For this review, take the finished solid that the model builds, in its own axes (mm). A direction names the side the tool comes from. Round coordinates to 2 decimals unless told otherwise and drop trailing zeros. Write each loop counter-clockwise with the first axis right and the second up, starting at its lowest first coordinate (ties: lowest second). Pieces come first, ordered by that corner, then holes. Notation, with made-up numbers: M -21.75,-24.75 L 37.25,-24.75 A26 ccw 37.25,4.25 Z; hole C 26,53 d5. An arc over 180 degrees is marked long. Answer in a Markdown table with one row per item.
```python
from build123d import *

# Parameters (mm, degrees)
MAIN_BODY_DEPTH          = 2.6
SKETCH4_W                = 17
SKETCH4_H                = 2.5
FLANGES_DEPTH            = 20.5
SKETCH5_R                = 2
DRILL_HOLD_EXTRUDE_DEPTH = 1.4
SKETCH2_R                = 3.2
SKETCH2_R_2              = 3.15
SKETCH2_R_3              = 1.5
SKETCH2_R_4              = 2.55
SCREW_HOLES_DEPTH        = 21.5
SCREW_HOLES_DEPTH_BACK   = 3.6
FLANGE_FILLET_R          = 2
SKETCH6_W                = 1.5
SKETCH6_H                = 11
FLANGE_NOTCHES_DEPTH     = 26
MAIN_LOWER_BODY_FILLET_R = 2


with BuildPart() as part:
    # Sketch1 → Main Body (new body)
    with BuildSketch(Plane(origin=(0, 0, 0), x_dir=(1, 0, 0), z_dir=(0, 1, 0))):
        with BuildLine():
            Line((11.7, -23.5), (32, -23.5))
            Line((32, -23.5), (32, 13.5))
            ThreePointArc((32, 13.5), (29.071067812, 20.571067812), (22, 23.5))
            Line((22, 23.5), (-22, 23.5))
            ThreePointArc((-22, 23.5), (-29.071067812, 20.571067812), (-32, 13.5))
            Line((-32, 13.5), (-32, -23.5))
            Line((-32, -23.5), (-12, -23.5))
            Line((-12, -23.5), (-12, -46))
            Line((-12, -46), (11.7, -46))
            Line((11.7, -46), (11.7, -23.5))
        make_face()
    extrude(amount=MAIN_BODY_DEPTH)

    # Sketch4 → Flanges (add)
    with BuildSketch(Plane(origin=(0, 2.6, 0), x_dir=(1, 0, 0), z_dir=(0, 1, 0))):
        with Locations((-23.5, -22.25)):
            Rectangle(SKETCH4_W, SKETCH4_H)
        with Locations((23.5, -22.25)):
            Rectangle(SKETCH4_W, SKETCH4_H)
    extrude(amount=FLANGES_DEPTH)

    # Sketch5 → Drill hold extrude (add)
    with BuildSketch(Plane(origin=(0, 2.6, 0), x_dir=(1, 0, 0), z_dir=(0, 1, 0))):
        with Locations((19, -9.3)):
            Circle(SKETCH5_R)
        with Locations((1.5, 9.3)):
            Circle(SKETCH5_R)
    extrude(amount=DRILL_HOLD_EXTRUDE_DEPTH)

    # Sketch2 → Screw holes (cut, two sides)
    with BuildSketch(Plane(origin=(0, 2.6, 0), x_dir=(1, 0, 0), z_dir=(0, 1, 0))) as screw_holes_sk:
        with Locations((-20.1, 15.8)):
            Circle(SKETCH2_R)
        with Locations((20, 16)):
            Circle(SKETCH2_R_2)
        with Locations((1.5, 9.3)):
            Circle(SKETCH2_R_3)
        with Locations((-23.6, -0.5)):
            Circle(SKETCH2_R_3)
        with Locations((-9.5, -0.5)):
            Circle(SKETCH2_R_3)
        with Locations((19, -9.3)):
            Circle(SKETCH2_R_3)
        with Locations((0.7, -31.3)):
            Circle(SKETCH2_R_4)
    extrude(amount=SCREW_HOLES_DEPTH, mode=Mode.SUBTRACT)
    extrude(screw_holes_sk.sketch, amount=-SCREW_HOLES_DEPTH_BACK, mode=Mode.SUBTRACT)

    # Flange Fillet
    flange_fillet_edges = [part.edges().sort_by_distance(p)[0] for p in [
        (-32, 23.1, 22.25),
        (-15, 23.1, 22.25),
        (32, 23.1, 22.25),
        (15, 23.1, 22.25),
    ]]
    fillet(flange_fillet_edges, radius=FLANGE_FILLET_R)

    # Sketch6 → Flange Notches (cut, through all)
    with BuildSketch(Plane(origin=(0, 0, 21), x_dir=(-1, 0, 0), z_dir=(0, 0, -1))):
        with Locations((-20.75, 17.6)):
            Rectangle(SKETCH6_W, SKETCH6_H)
        with Locations((20.75, 17.6)):
            Rectangle(SKETCH6_W, SKETCH6_H)
    extrude(amount=-FLANGE_NOTCHES_DEPTH, mode=Mode.SUBTRACT)

    # Main lower body Fillet
    main_lower_body_fillet_edges = [part.edges().sort_by_distance(p)[0] for p in [
        (11.7, 1.3, 46),
        (-12, 1.3, 46),
    ]]
    fillet(main_lower_body_fillet_edges, radius=MAIN_LOWER_BODY_FILLET_R)


solid = part.part
```
Q1. Machinability: for faces 5 (the face through (17.526, 3.29, 7.948)), 6 (the face through (11.7, 1, 34)), 7 (the face through (21.5, 18, 22)), 8 (the face through (1.175, 2.028, -7.836)), which of the approach directions +Z, -Z, +X, -X, +Y, -Y give a long, thin tool a straight path to every point of the face, cutting with its end or side? Answer none if there is none.
Found:
| item | result |
|---|---|
| face 5 | +Y |
| face 6 | +Z, +X, +Y, -Y |
| face 7 | +Z, -Z, +Y |
| face 8 | +Y, -Y |
Q2. Take a section at A-A (y = 8.25). State the section outline as (x, z) points, then the cut area to 3 significant figures.
Found:
| item | result |
|---|---|
| outline | M -32,21 L -15,21 L -15,23.5 L -32,23.5 Z; M 15,21 L 32,21 L 32,23.5 L 15,23.5 Z |
| area | 85.0 mm² |
Q3. Take a section at B-B (y = 18). State the section outline as (x, z) points, then the cut area to 3 significant figures.
Found:
| item | result |
|---|---|
| outline | M -32,21 L -21.5,21 L -21.5,23.5 L -32,23.5 Z; M -20,21 L -15,21 L -15,23.5 L -20,23.5 Z; M 15,21 L 20,21 L 20,23.5 L 15,23.5 Z; M 21.5,21 L 32,21 L 32,23.5 L 21.5,23.5 Z |
| area | 77.5 mm² |
Q4. For probe 1 along Z at (x, y) = (19, 3.05); probe 2 along X at (y, z) = (2, 0.5); probe 3 along Z at (x, y) = (1.5, 2.85), list the stretches that pass through material, from the lowest coordinate up.
Found:
| item | result |
|---|---|
| probe 1 | 7.3 to 7.8, 10.8 to 11.3, 21 to 23.5 |
| probe 2 | -32 to -25.1, -22.1 to -11, -8 to 32 |
| probe 3 | -11.3 to -10.8, -7.8 to -7.3 |
Q5. Take a section at D-D (x = 19). State the section outline as (y, z) points, then the cut area to 3 significant figures.
Found:
| item | result |
|---|---|
| outline | M 0,-23.5 L 2.6,-23.5 L 2.6,-18.99 L 0,-18.99 Z; M 0,-13.01 L 2.6,-13.01 L 2.6,7.3 L 4,7.3 L 4,7.8 L 0,7.8 Z; M 0,10.8 L 4,10.8 L 4,11.3 L 2.6,11.3 L 2.6,21 L 23.1,21 L 23.1,23.5 L 0,23.5 Z |
| area | 152 mm² |
Q6. Mouldability with a two-part tool opening along Z and no side actions: class faces 1 (the face through (29.15, 1.28, -20.49)), 2 (the face through (-17.048, 1.318, -16.761)), 3 (the face through (1.066, 3.29, -7.348)), 4 (the face through (31.43, 22.5, 22.23)) as +Z half, -Z half, draft (parallel to the pull), parting line (faces both ways), or undercut.
Found:
| item | result |
|---|---|
| face 1 | -Z half |
| face 2 | undercut |
| face 3 | parting line |
| face 4 | draft |
Q7. Insertion check: P1, Ø13.5, axis at x = -21, y = 11.5, coming from the -Z side; P2, Ø6, axis at x = -19, y = 7.5, coming from the +Z side; P3, Ø12, axis at x = -12.5, y = 7.5, coming from the +Z side; P4, Ø0.8, axis at y = 1, z = 38.5, coming from the +X side. Each pin has a flat end and moves straight along its axis. Give the tip position at first contact, or say it passes through.
Found:
| item | result |
|---|---|
| P1 | z = 21 |
| P2 | z = 23.5 |
| P3 | z = 46 |
| P4 | x = 11.7 |
Q8. Take a section at C-C (z = 31.3). State the section outline as (x, y) points, then the cut area to 3 significant figures.
Found:
| item | result |
|---|---|
| outline | M -12,0 L -1.85,0 L -1.85,2.6 L -12,2.6 Z; M 3.25,0 L 11.7,0 L 11.7,2.6 L 3.25,2.6 Z |
| area | 48.4 mm² |
